Part model, mm, in its own coordinate system. A direction names the side the tool comes from. Give positions to 0.01 mm unless a question says otherwise; leave off trailing zeros. Write each loop counter-clockwise with the first axis right and the second up, starting at its lowest first coordinate (ties: lowest second). Pieces come first, ordered by that corner, then holes. Notation, with made-up numbers: M -25.75,88 L 7.25,88 A23 cw 7.25,114 Z; hole C 18.25,19.25 d4. An arc over 180 degrees is marked long. Answer as CSV lines item,"result". Start each with the question number.
1) Slice it at B-B, the plane z = 6.25. Give the cut face in (x, y).
2) Pin check, flat tips, straight feed: pin 1 Ø5 at (x, y) = (-1, -5.5) entering from -Z; pin 2 Ø4 at (y, z) = (-3, 2.5) entering from +X; pin 3 Ø2 at (y, z) = (4, 7) entering from +X; pin 4 Ø3 at (y, z) = (2.5, 3.5) entering from -X. Stop position of each tip, or through.
3) Slice it at D-D, the plane z = 1. Give the cut face in (x, y), plus the area to 3 significant figures.
4) Slice it at A-A, the plane x = 0. Give the cut face in (y, z), plus the area to 3 significant figures.
5) Wall check: line 1 along Y through (x, z) = (-3.25, 2); line 2 along X through (y, z) = (3.75, 2.75); line 3 along X through (y, z) = (-1.5, 0.5). Give the ranges that are in metal, low to high. Write a range as from..to.
6) Mould opens along Y. For faces 1 (the cylindrical face through (0, 6.2, 5.4)), 2 (the flat face through (0, 0, 9)), 3 (the flat face through (-4.7, -4.7, 2)) say: pulls with the +Y half, pulls with the -Y half, needs draft (parallel to the pull), parting line crosses it, or undercut.
7) Tool access for faces 4 (the cylindrical face through (4.37, 4.4, 5.35)), 5 (the cylindrical face through (-6.2, 0, 5.4)), 6 (the cylindrical face through (6.2, 0, 5.4)), 7 (the cylindrical face through (0, -6.2, 5.4)): list every direction of +Z, -Z, +X, -X, +Y, -Y with a clear straight run to the whole face (end or side of a thin tool).
```python
from build123d import *

# Parameters (mm, degrees)
CYLINDER001_R     = 0.8
CYLINDER001_DEPTH = 10
ARRAY_COUNT       = 8
CYLINDER_R        = 7
CYLINDER_DEPTH    = 9
CHAMFER_SIZE      = 1


with BuildPart() as array:
    # Cylinder001 → Cylinder001 (new body)
    with BuildSketch(Plane(origin=(7, 0, 0), x_dir=(1, 0, 0), z_dir=(0, 0, 1))):
        Circle(CYLINDER001_R)
    extrude(amount=CYLINDER001_DEPTH)

    # Array: Array ×8 about axis
    array_axis = Axis((0, 0, 0), (0, 0, 1))


with BuildPart() as array_1:
    add(array.part)
    for i in range(1, ARRAY_COUNT):
        add(array.part.rotate(array_axis, i * 360 / ARRAY_COUNT))


with BuildPart() as array_2:
    # Array placement: moved
    add(array_1.part.moved(Location((0, 0, 2))))


with BuildPart() as cut:
    # Cylinder → Cylinder (new body)
    with BuildSketch(Plane.XY):
        Circle(CYLINDER_R)
    extrude(amount=CYLINDER_DEPTH)

    # Chamfer
    chamfer_edges = [cut.edges().sort_by_distance(p)[0] for p in [
        (-7, 0, 9),
    ]]
    chamfer(chamfer_edges, length=CHAMFER_SIZE)

    # Cut: cut Array
    add(array_2.part, mode=Mode.SUBTRACT)


solid = cut.part
```
Found:
1,outline,"M -6.95,-0.8 A7 ccw -5.48,-4.35 A0.8 cw -4.35,-5.48 A7 ccw -0.8,-6.95 A0.8 cw 0.8,-6.95 A7 ccw 4.35,-5.48 A0.8 cw 5.48,-4.35 A7 ccw 6.95,-0.8 A0.8 cw 6.95,0.8 A7 ccw 5.48,4.35 A0.8 cw 4.35,5.48 A7 ccw 0.8,6.95 A0.8 cw -0.8,6.95 A7 ccw -4.35,5.48 A0.8 cw -5.48,4.35 A7 ccw -6.95,0.8 A0.8 cw Z"
2,pin 1,"z = 0"
2,pin 2,"x = 6.93"
2,pin 3,"x = 6.32"
2,pin 4,"x = -6.93"
3,outline,"C 0,0 d14"
3,area,"154 mm²"
4,outline,"M -7,0 L 7,0 L 7,2 L 6.2,2 L 6.2,8.8 L 6,9 L -6,9 L -6.2,8.8 L -6.2,2 L -7,2 Z"
4,area,"115 mm²"
5,line 1,"-6.2..6.2"
5,line 2,"-5.91..5.91"
5,line 3,"-6.84..6.84"
6,face 1,"pulls with the +Y half"
6,face 2,"needs draft"
6,face 3,"undercut"
7,face 4,"+Z"
7,face 5,"+Z, -X"
7,face 6,"+Z, +X"
7,face 7,"+Z, -Y"
